```python
from build123d import *

# Parameters (mm, degrees)
SHELL1_T = -2.54


with BuildPart() as part:
    # Sketch1 → Revolve2 (revolve)
    with BuildSketch(Plane(origin=(0, 0, 0), x_dir=(1, 0, 0), z_dir=(0, 1, 0))):
        Polygon((0, 0), (0, 25.273), (50.8, 25.273), (50.8, 28.194), (209.55, 0), align=None)
    revolve(axis=Axis((0, 0, 0), (1, 0, 0)))

    # Shell1
    shell1_openings = [part.faces().sort_by_distance(p)[0] for p in [
        (0, 0, 25.273),
    ]]
    offset(amount=SHELL1_T, openings=shell1_openings, kind=Kind.INTERSECTION)


solid = part.part
```
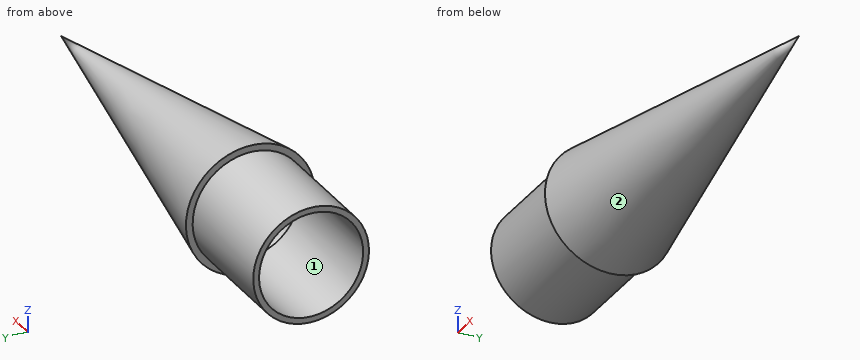
For this review, take the finished solid that the model builds, in its own axes (mm). Face numbers are marked on the shaded views. Give positions to 0.01 mm unless a question says otherwise; leave off trailing zeros. Write each loop counter-clockwise with the first axis right and the second up, starting at its lowest first coordinate (ties: lowest second). Pieces come first, ordered by that corner, then holes. Notation, with made-up numbers: M 20,39 L 63,39 A15 cw 63,64 Z; hole C 61.5,-12.75 d1. An arc over 180 degrees is marked long. Answer as a JSON object with one key per item and string values. Group by question number.
Item 1: Consider section B-B on x = 102.5. Write out the cut boundary in (y, z), plus the area to 3 significant figures.
Item 2: For pin 1 Ø8 at (x, z) = (25.5, -2) entering from -Y; pin 2 Ø1.5 at (x, y) = (79.5, 2.5) entering from +Z; pin 3 Ø10 at (x, z) = (89, -20) entering from +Y; pin 4 Ø15 at (y, z) = (-4.5, 4.5) entering from +X, all flat-tipped, find the tip position at first contact; note any pin that passes through.
Item 3: For probe 1 along Z at (x, y) = (21.5, -15); probe 2 along Y at (x, z) = (35, 0); probe 3 along Y at (x, z) = (146.5, 5.5), list the stretches that pass through material, from the lowest coordinate up. Write a range as [from, to].
Item 4: Consider section A-A on x = 14. Write out the cut boundary in (y, z).
Item 5: Draft analysis for pull direction Y (two halves, no side actions). For the marked faces 1 and 2, state which applies: +Y half, -Y half, draft (parallel to the pull), parting line (faces both ways), or undercut.
Check result:
{
 "1": {"outline": "C 0,0 d38.02; hole C 0,0 d32.86", "area": "287 mm^2"},
 "2": {"pin 1": "stops at y = -25.27", "pin 2": "stops at z = 23.11", "pin 3": "stops at y = 15.43", "pin 4": "stops at x = 209.55"},
 "3": {"probe 1": "z = [-20.34, -17.08], [17.08, 20.34]", "probe 2": "y = [-25.27, -22.73], [22.73, 25.27]", "probe 3": "y = [-9.75, -6.63], [6.63, 9.75]"},
 "4": {"outline": "C 0,0 d50.55; hole C 0,0 d45.47"},
 "5": {"face 1": "undercut", "face 2": "parting line"}
}
